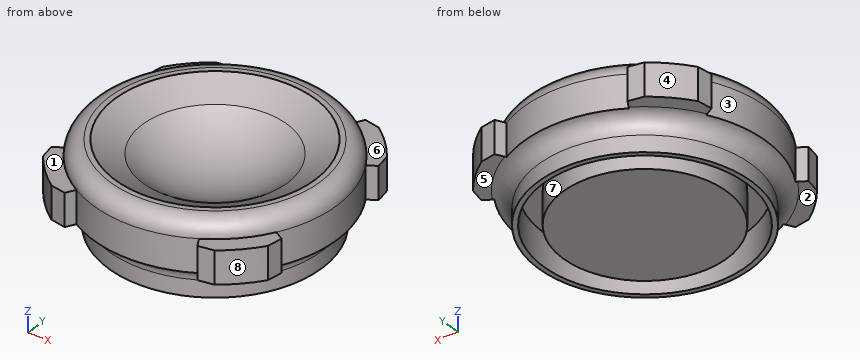
from build123d import *

# Parameters (mm, degrees)
SKETCH_1_R                           = 37
EXTRUDE_1_DEPTH                      = 15
FILLET_2_R                           = 5
EXTRUDE_3_DEPTH                      = 10
CHAMFER_2_SIZE                       = 1.819851171
CHAMFER_3_SIZE                       = 1.819851171
PATTERN_CIRCULAR_4_COUNT             = 4
CHAMFER_2_OF_PATTERN_CIRCULAR_4_SIZE = 1.819851171
CHAMFER_3_OF_PATTERN_CIRCULAR_4_SIZE = 1.819851171
SKETCH_9_R                           = 32.5
SKETCH_9_R_2                         = 31
EXTRUDE_4_DEPTH                      = 10
SKETCH_9_3_R                         = 25
EXTRUDE_5_DEPTH                      = 10
FILLET_3_R                           = 5


with BuildPart() as part:
    # 草圖1 → 填料-伸長1 (new body)
    with BuildSketch(Plane.XY):
        Circle(SKETCH_1_R)
    extrude(amount=EXTRUDE_1_DEPTH)

    # 草圖2 → 除料-旋轉2 (revolve, cut)
    with BuildSketch(Plane.XY.offset(38)):
        with BuildLine():
            Line((-35, 0), (35, 0))
            ThreePointArc((35, 0), (0, -35), (-35, 0))
        make_face()
    revolve(axis=Axis((-35, 0, 38), (1, 0, 0)), mode=Mode.SUBTRACT)

    # 導角1: read off the stored shape, not the designer's step
    # 導角1 outline → 導角1 (revolve, cut)
    with BuildSketch(Plane.XZ):
        Polygon((22.017739237, 15), (22.017739237, 10.79303106), (30.419689063, 15), align=None)
    revolve(axis=Axis((0, 0, 0), (0, 0, 1)), mode=Mode.SUBTRACT)

    # 圓角2
    fillet_2_edges = [part.edges().sort_by_distance(p)[0] for p in [
        (-37, 0, 15),
    ]]
    fillet(fillet_2_edges, radius=FILLET_2_R)

    # 草圖8 → 填料-伸長3 (add)
    with BuildSketch(Plane.XY):
        with BuildLine():
            Line((21, 36.373066959), (18.5, 32.04293994))
            ThreePointArc((18.5, 32.04293994), (26.162950904, 26.162950904), (32.04293994, 18.5))
            Line((32.04293994, 18.5), (36.373066959, 21))
            ThreePointArc((36.373066959, 21), (29.69848481, 29.69848481), (21, 36.373066959))
        make_face()
    extrude_3 = extrude(amount=EXTRUDE_3_DEPTH)

    # 導角2
    # the kernel refuses this chamfer: 5, 1.819851171 mm, written as the material it takes off along each edge
    with BuildSketch(Plane(origin=(21, 36.373066959, -11.408988882), x_dir=(-0.5000000000000003, -0.8660254037844385, 0), z_dir=(0, 0, 1))) as chamfer_2_piece_1:
        with BuildLine():
            Line((CHAMFER_2_SIZE, 0), (0.22826162, 4.372856354))
            ThreePointArc((0.22826162, 4.372856354), (0.06200601, 2.281372415), (0, 0))
            Line((0, 0), (CHAMFER_2_SIZE, 0))
        make_face()
    extrude(amount=32.817977764, mode=Mode.SUBTRACT)

    # 導角3
    # the kernel refuses this chamfer: 5, 1.819851171 mm, written as the material it takes off along each edge
    with BuildSketch(Plane(origin=(36.373066959, 21, -11.408988882), x_dir=(-0.8660254037844387, -0.5000000000000001, 0), z_dir=(0, 0, 1))) as chamfer_3_piece_1:
        with BuildLine():
            Line((CHAMFER_3_SIZE, 0), (0.22826162, -4.372856354))
            ThreePointArc((0.22826162, -4.372856354), (0.06200601, -2.281372415), (0, 0))
            Line((0, 0), (CHAMFER_3_SIZE, 0))
        make_face()
    extrude(amount=32.817977764, mode=Mode.SUBTRACT)

    # 環狀複製排列4: 填料-伸長3 ×4 about axis
    pattern_circular_4_axis = Axis((0, 0, 0), (0, 0, 1))
    for i in range(1, PATTERN_CIRCULAR_4_COUNT):
        add(extrude_3.rotate(pattern_circular_4_axis, i * 360 / PATTERN_CIRCULAR_4_COUNT))

    # 導角2 of 環狀複製排列4
    # the kernel refuses this chamfer: 5, 1.819851171 mm, written as the material it takes off along each edge
    with BuildSketch(Plane(origin=(-36.373066959, 21, -11.408988882), x_dir=(0.5444649568890038, 0.8387835899204604, 0), z_dir=(0, 0, 1)), Plane(origin=(-21, -36.373066959, -11.408988882), x_dir=(-0.8387835899204604, 0.5444649568890038, 0), z_dir=(0, 0, 1)), Plane(origin=(36.373066959, -21, -11.408988882), x_dir=(-0.5444649568890034, -0.8387835899204606, 0), z_dir=(0, 0, 1))) as chamfer_2_of_pattern_circular_4_piece_1:
        with BuildLine():
            Line((4.378809891, 0), (CHAMFER_2_OF_PATTERN_CIRCULAR_4_SIZE * 0.0521286891855, -CHAMFER_2_OF_PATTERN_CIRCULAR_4_SIZE * 0.998640375775))
            Line((CHAMFER_2_OF_PATTERN_CIRCULAR_4_SIZE * 0.0521286891855, -CHAMFER_2_OF_PATTERN_CIRCULAR_4_SIZE * 0.998640375775), (0, 0))
            ThreePointArc((0, 0), (2.281502898, 0.057003248), (4.378809891, 0))
        make_face()
    extrude(amount=32.817977764, mode=Mode.SUBTRACT)

    # 導角3 of 環狀複製排列4
    # the kernel refuses this chamfer: 5, 1.819851171 mm, written as the material it takes off along each edge
    with BuildSketch(Plane(origin=(-21, 36.373066959, -11.408988882), x_dir=(0.5000000000000001, -0.8660254037844387, 0), z_dir=(0, 0, 1))) as chamfer_3_of_pattern_circular_4_piece_1:
        with BuildLine():
            Line((CHAMFER_3_OF_PATTERN_CIRCULAR_4_SIZE, 0), (0.22826162, -4.372856354))
            ThreePointArc((0.22826162, -4.372856354), (0.06200601, -2.281372415), (0, 0))
            Line((0, 0), (CHAMFER_3_OF_PATTERN_CIRCULAR_4_SIZE, 0))
        make_face()
    extrude(amount=32.817977764, mode=Mode.SUBTRACT)
    with BuildSketch(Plane(origin=(-36.373066959, -21, -11.408988882), x_dir=(0.5444649568890013, -0.8387835899204622, 0), z_dir=(0, 0, 1)), Plane(origin=(21, -36.373066959, -11.408988882), x_dir=(0.8387835899204622, 0.5444649568890012, 0), z_dir=(0, 0, 1))) as chamfer_3_of_pattern_circular_4_piece_2:
        with BuildLine():
            Line((4.378809891, 0), (CHAMFER_3_OF_PATTERN_CIRCULAR_4_SIZE * 0.0521286891855, CHAMFER_3_OF_PATTERN_CIRCULAR_4_SIZE * 0.998640375775))
            Line((CHAMFER_3_OF_PATTERN_CIRCULAR_4_SIZE * 0.0521286891855, CHAMFER_3_OF_PATTERN_CIRCULAR_4_SIZE * 0.998640375775), (0, 0))
            ThreePointArc((0, 0), (2.281502898, -0.057003248), (4.378809891, 0))
        make_face()
    extrude(amount=32.817977764, mode=Mode.SUBTRACT)

    # 草圖9 → 填料-伸長4 (add)
    with BuildSketch(Plane(origin=(0, 0, 0), x_dir=(-1, 0, 0), z_dir=(0, 0, -1))):
        with Locations(Location((0, 0, 0), (0, 0, 180))):
            Circle(SKETCH_9_R)
        Circle(SKETCH_9_R_2, mode=Mode.SUBTRACT)
    extrude(amount=EXTRUDE_4_DEPTH)

    # 草圖9<3> → 填料-伸長5 (add)
    with BuildSketch(Plane(origin=(0, 0, 0), x_dir=(-1, 0, 0), z_dir=(0, 0, -1))):
        with Locations(Location((0, 0, 0), (0, 0, 180))):
            Circle(SKETCH_9_3_R)
    extrude(amount=EXTRUDE_5_DEPTH)

    # 圓角3
    # the kernel refuses this fillet: 5 mm, written as the material it adds along each edge
    with BuildSketch(Plane(origin=(0, 0, 0), x_dir=(1, 0, 0), z_dir=(0, 1, 0))) as fillet_3_piece_1_section:
        with BuildLine():
            CenterArc((32.5 + FILLET_3_R, FILLET_3_R), FILLET_3_R, 180, 90)
            Line((32.5, FILLET_3_R), (32.5, 0))
            Line((32.5, 0), (32.5 + FILLET_3_R, 0))
        make_face()
    fillet_3_piece_1 = revolve(axis=Axis((0, 0, 0), (0, 0, -1)), mode=Mode.PRIVATE)
    fillet_3_piece_1 = fillet_3_piece_1 & Plane(origin=(0, 0, 0), x_dir=(1, 0, 0), z_dir=(0, 0, -1)) * Cylinder(37, 150, mode=Mode.PRIVATE)
    add(fillet_3_piece_1)
    with BuildSketch(Plane(origin=(0, 0, 0), x_dir=(1, 0, 0), z_dir=(0, 1, 0))) as fillet_3_piece_2_section:
        with BuildLine():
            CenterArc((32.5 + FILLET_3_R, FILLET_3_R), FILLET_3_R, 180, 90)
            Line((32.5, FILLET_3_R), (32.5, 0))
            Line((32.5, 0), (32.5 + FILLET_3_R, 0))
        make_face()
    fillet_3_piece_2 = revolve(axis=Axis((0, 0, 0), (0, 0, -1)), mode=Mode.PRIVATE)
    fillet_3_piece_2 = split(fillet_3_piece_2, bisect_by=Plane(origin=(0, 0, 0), z_dir=(0.8660254037844387, 0.5000000000000001, 0)), keep=Keep.TOP, mode=Mode.PRIVATE)
    fillet_3_piece_2 = split(fillet_3_piece_2, bisect_by=Plane(origin=(0, 0, 0), z_dir=(-0.4999999999999997, -0.8660254037844389, 0)), keep=Keep.TOP, mode=Mode.PRIVATE)
    add(fillet_3_piece_2)
    with BuildSketch(Plane(origin=(0, 0, 0), x_dir=(1, 0, 0), z_dir=(0, 1, 0))) as fillet_3_piece_3_section:
        with BuildLine():
            CenterArc((32.5 + FILLET_3_R, FILLET_3_R), FILLET_3_R, 180, 90)
            Line((32.5, FILLET_3_R), (32.5, 0))
            Line((32.5, 0), (32.5 + FILLET_3_R, 0))
        make_face()
    fillet_3_piece_3 = revolve(axis=Axis((0, 0, 0), (0, 0, -1)), mode=Mode.PRIVATE)
    fillet_3_piece_3 = split(fillet_3_piece_3, bisect_by=Plane(origin=(0, 0, 0), z_dir=(0.8660254037844388, -0.4999999999999997, 0)), keep=Keep.TOP, mode=Mode.PRIVATE)
    fillet_3_piece_3 = split(fillet_3_piece_3, bisect_by=Plane(origin=(0, 0, 0), z_dir=(-0.5000000000000001, 0.8660254037844386, 0)), keep=Keep.TOP, mode=Mode.PRIVATE)
    add(fillet_3_piece_3)
    with BuildSketch(Plane(origin=(0, 0, 0), x_dir=(1, 0, 0), z_dir=(0, 1, 0))) as fillet_3_piece_4_section:
        with BuildLine():
            CenterArc((32.5 + FILLET_3_R, FILLET_3_R), FILLET_3_R, 180, 90)
            Line((32.5, FILLET_3_R), (32.5, 0))
            Line((32.5, 0), (32.5 + FILLET_3_R, 0))
        make_face()
    fillet_3_piece_4 = revolve(axis=Axis((0, 0, 0), (0, 0, -1)), mode=Mode.PRIVATE)
    fillet_3_piece_4 = split(fillet_3_piece_4, bisect_by=Plane(origin=(0, 0, 0), z_dir=(-0.8660254037844388, 0.4999999999999997, 0)), keep=Keep.TOP, mode=Mode.PRIVATE)
    fillet_3_piece_4 = split(fillet_3_piece_4, bisect_by=Plane(origin=(0, 0, 0), z_dir=(0.5000000000000001, -0.8660254037844386, 0)), keep=Keep.TOP, mode=Mode.PRIVATE)
    add(fillet_3_piece_4)
    with BuildSketch(Plane(origin=(0, 0, 0), x_dir=(1, 0, 0), z_dir=(0, 1, 0))) as fillet_3_piece_5_section:
        with BuildLine():
            CenterArc((32.5 + FILLET_3_R, FILLET_3_R), FILLET_3_R, 180, 90)
            Line((32.5, FILLET_3_R), (32.5, 0))
            Line((32.5, 0), (32.5 + FILLET_3_R, 0))
        make_face()
    fillet_3_piece_5 = revolve(axis=Axis((0, 0, 0), (0, 0, -1)), mode=Mode.PRIVATE)
    fillet_3_piece_5 = split(fillet_3_piece_5, bisect_by=Plane(origin=(0, 0, 0), z_dir=(-0.8660254037844387, -0.5000000000000001, 0)), keep=Keep.TOP, mode=Mode.PRIVATE)
    fillet_3_piece_5 = split(fillet_3_piece_5, bisect_by=Plane(origin=(0, 0, 0), z_dir=(0.4999999999999997, 0.8660254037844389, 0)), keep=Keep.TOP, mode=Mode.PRIVATE)
    add(fillet_3_piece_5)


solid = part.part
Build history of the part. All positions in model axes, mm. Face numbers are marked on the shaded views. A direction names the side the tool comes from. Round coordinates to 2 decimals unless told otherwise and drop trailing zeros. Write each loop counter-clockwise with the first axis right and the second up, starting at its lowest first coordinate (ties: lowest second). Pieces come first, ordered by that corner, then holes. Notation, with made-up numbers: M -33.75,-9 L 8.25,-9 A20 cw 8.25,21 Z; hole C 63,1 d4. An arc over 180 degrees is marked long. Answer as a JSON object with one key per item and string values. Group by question number.
(1) Which spindle directions (+Z, -Z, +X, -X, +Y, -Y) get a long thin tool onto all of the face, cutting with end or side? Do the marked faces 4, 5, 6, 7 and 8. Say none if no direction does.
(2) Flat gauge pins, fed straight in: pin 1 (13 mm diameter, centred on x = -28.5, y = -29.5, fed in from -Z); pin 2 (5 mm diameter, centred on x = 23.5, y = -30, fed in from -Z); pin 3 (5 mm diameter, centred on x = -24, y = 28, fed in from +Z). Where does each tip first touch, or does it go through?
(3) Drill centre lines: L1, parallel to Y at x = 0, z = -4.75; L2, parallel to X at y = 21, z = -6.5; L3, parallel to Y at x = 7, z = -3.5. Where is each one in solid material? Low to high.
(4) Cut at A-A (x = 0). Give the cut face in (y, z).
(5) Mould opens along Z. For the marked faces 1, 2 and 3 say: pulls with the +Z half, pulls with the -Z half, needs draft (parallel to the pull), parting line crosses it, or undercut.
Responses:
{
 "1": {"face 4": "+Z, -Z, -X, +Y", "face 5": "-Z, +X, +Y", "face 6": "+Z, +X, +Y", "face 7": "-Z", "face 8": "+Z, -Z, +X, -Y"},
 "2": {"pin 1": "stops at z = -0.99", "pin 2": "stops at z = -0.37", "pin 3": "stops at z = 14.4"},
 "3": {"L1": "y = -32.51 to -31, -25 to 25, 31 to 32.51", "L2": "x = -24.8 to -22.8, -13.56 to 13.56, 22.8 to 24.8", "L3": "y = -31.97 to -30.2, -24 to 24, 30.2 to 31.97"},
 "4": {"outline": "M -37,-0.03 A5 cw -32.5,-5 L -32.5,-10 L -31,-10 L -31,0 L -25,0 L -25,-10 L 25,-10 L 25,0 L 31,0 L 31,-10 L 32.5,-10 L 32.5,-5 A5 cw 37,-0.03 L 37,10 A5 ccw 32,15 L 30.42,15 L 22.02,10.79 A35 cw -22.02,10.79 L -30.42,15 L -32,15 A5 ccw -37,10 Z"},
 "5": {"face 1": "pulls with the +Z half", "face 2": "pulls with the -Z half", "face 3": "needs draft"}
}
